```python
from build123d import *

# Parameters (mm, degrees)
ESQUISSE1_W        = 12.3
ESQUISSE1_H        = 23.3
BOSS_EXTRU_1_DEPTH = 17
ESQUISSE2_W        = 12.3
ESQUISSE2_H        = 32.2
ESQUISSE2_R        = 1.25
BOSS_EXTRU_2_DEPTH = 2.5
ESQUISSE3_W        = 12.3
ESQUISSE3_H        = 23.3
BOSS_EXTRU_3_DEPTH = 4.3
BOSS_EXTRU_4_DEPTH = 4.3
ESQUISSE5_R        = 2.45
BOSS_EXTRU_5_DEPTH = 3.2


with BuildPart() as part:
    # Esquisse1 → Boss.-Extru.1 (new body)
    with BuildSketch(Plane.XY):
        with Locations((6.15, 11.65)):
            Rectangle(ESQUISSE1_W, ESQUISSE1_H)
    extrude(amount=BOSS_EXTRU_1_DEPTH)

    # Esquisse2 → Boss.-Extru.2 (add)
    with BuildSketch(Plane.XY.offset(17)):
        with Locations((6.15, 11.65)):
            Rectangle(ESQUISSE2_W, ESQUISSE2_H)
        with Locations((6.15, 25.4)):
            Circle(ESQUISSE2_R, mode=Mode.SUBTRACT)
        with Locations(Location((6.15, -2.1, 0), (0, 0, 180))):
            Circle(ESQUISSE2_R, mode=Mode.SUBTRACT)
    extrude(amount=BOSS_EXTRU_2_DEPTH)

    # Esquisse3 → Boss.-Extru.3 (add)
    with BuildSketch(Plane.XY.offset(19.5)):
        with Locations((6.15, 11.65)):
            Rectangle(ESQUISSE3_W, ESQUISSE3_H)
    extrude(amount=BOSS_EXTRU_3_DEPTH)

    # Esquisse4 → Boss.-Extru.4 (add)
    with BuildSketch(Plane.XY.offset(23.8)):
        with BuildLine():
            ThreePointArc((4.176616397, 11.974796748), (6.15, 0), (8.123383603, 11.974796748))
            ThreePointArc((8.123383603, 11.974796748), (6.15, 14.3), (4.176616397, 11.974796748))
        make_face()
    extrude(amount=BOSS_EXTRU_4_DEPTH)

    # Esquisse5 → Boss.-Extru.5 (add)
    with BuildSketch(Plane.XY.offset(28.1)):
        with Locations((6.15, 6.15)):
            Circle(ESQUISSE5_R)
    extrude(amount=BOSS_EXTRU_5_DEPTH)


solid = part.part
```
For this review, take the finished solid that the model builds, in its own axes (mm). A direction names the side the tool comes from. Round coordinates to 2 decimals unless told otherwise and drop trailing zeros. Write each loop counter-clockwise with the first axis right and the second up, starting at its lowest first coordinate (ties: lowest second). Pieces come first, ordered by that corner, then holes. Notation, with made-up numbers: (-4.75, 70) - (9.25, 70) arc R18 ccw to (9.25, 90) - close; hole circle Ø3 at (34, -38.75). An arc over 180 degrees is marked (long way). Answer as a JSON object with one key per item and string values.
1. We need section B-B on z = 17.5. Give the boundary of the cut face in (x, y), then the cut area to 3 significant figures.
Response values:
{"outline": "(0, -4.45) - (12.3, -4.45) - (12.3, 27.75) - (0, 27.75) - close; hole circle Ø2.5 at (6.15, -2.1); hole circle Ø2.5 at (6.15, 25.4)", "area": "386 mm2"}
2. For pin 1 Ø1.5 at (x, z) = (4, 25.5) entering from -Y; pin 2 Ø6 at (x, z) = (2.5, 8) entering from +Y; pin 3 Ø3.5 at (x, y) = (8, 25) entering from +Z; pin 4 Ø2 at (x, y) = (6.15, 25.4) entering from +Z, all flat-tipped, find the tip position at first contact; note any pin that passes through.
Response values:
{"pin 1": "stops at y = 0.16", "pin 2": "stops at y = 23.3", "pin 3": "stops at z = 23.8", "pin 4": "passes through"}
3. Draft analysis for pull direction X (two halves, no side actions). For faces 6 (the face through (6, 23.3, 22)), 7 (the face through (5.229, 26.245, 18.232)), 8 (the face through (12.3, 11, 12)), 9 (the face through (6.42, -0.88, 18.23)), state which applies: +X half, -X half, draft (parallel to the pull), parting line (faces both ways), or undercut.
Response values:
{"face 6": "draft", "face 7": "undercut", "face 8": "+X half", "face 9": "undercut"}
4. To check wall thickness, follow line 1 along Y through (x, z) = (6.15, 18.25); line 2 along Z through (x, y) = (6, 9.5); line 3 along X through (y, z) = (-2, 18). State the ranges of each line that lie inside material, in increasing order.
Response values:
{"line 1": "y = -4.45 to -3.35, -0.85 to 24.15, 26.65 to 27.75", "line 2": "z = 0 to 28.1", "line 3": "x = 0 to 4.9, 7.4 to 12.3"}
5. We need section C-C on x = 5.5. Count the separate pieces of the cut face and the enclosed holes in it, then the cut area to 3 significant figures.
Response values:
{"separate pieces": "3", "enclosed holes": "0", "area": "642 mm2"}
6. We need section A-A on y = 25.4. Give the boundary of the cut face in (x, z), then the cut area to 3 significant figures.
Response values:
{"outline": "(0, 17) - (4.9, 17) - (4.9, 19.5) - (0, 19.5) - close; (7.4, 17) - (12.3, 17) - (12.3, 19.5) - (7.4, 19.5) - close", "area": "24.5 mm2"}
7. Tool access review of faces 1 (the face through (4.7, 25.6, 19.5)), 2 (the face through (4.7, 25.6, 17)), 3 (the face through (11, 1, 23.8)), 4 (the face through (6, 0, 8)), 5 (the face through (5.62, 3.76, 29.68)): name each direction out of +Z, -Z, +X, -X, +Y, -Y from which nothing blocks a thin tool from reaching the whole face with its end or side.
Response values:
{"face 1": "+Z, +X, -X, +Y", "face 2": "-Z, +X, -X, +Y", "face 3": "+Z, +X, -Y", "face 4": "-Z, +X, -X, -Y", "face 5": "+Z"}
8. We need section D-D on x = 0.75. Give the boundary of the cut face in (y, z).
Response values:
{"outline": "(-4.45, 17) - (0, 17) - (0, 0) - (23.3, 0) - (23.3, 17) - (27.75, 17) - (27.75, 19.5) - (23.3, 19.5) - (23.3, 23.8) - (9.09, 23.8) - (9.09, 28.1) - (3.21, 28.1) - (3.21, 23.8) - (0, 23.8) - (0, 19.5) - (-4.45, 19.5) - close"}
